The model under review builds one solid part; all positions refer to its coordinate system, in mm. A direction names the side the tool comes from. Coordinates: 2 decimals unless noted, no trailing zeros. Loops run counter-clockwise (first coordinate to the right, second up) from the corner with the lowest first, then second, coordinate; pieces in that order, holes last. Notation, with made-up numbers: (18, -4) - (54, -4) arc R17 ccw to (54, 28) - close; hole circle Ø11 at (-2.75, 30.25). An arc over 180 degrees is marked (long way). Answer in a Markdown table with one row per item. Add a question column.
(1) We need section B-B on y = 0.45. Write out the cut boundary in (x, z), plus the area to 3 significant figures.
(2) Mouldability with a two-part tool opening along X and no side actions: class faces 5 (the flat face through (20.41, 0.02, 18.64)), 6 (the flat face through (20.15, 3, -11)), 7 (the flat face through (0, -1.25, 0)) as +X half, -X half, draft (parallel to the pull), parting line (faces both ways), or undercut.
(3) We need section A-A on z = -8.7. Write out the cut boundary in (x, y), plus the area to 3 significant figures.
(4) Machinability: for faces 1 (the flat face through (15, 3, -12)), 2 (the flat face through (-16, 3, 14.5)), 3 (the flat face through (19, 3, -7)), 4 (the flat face through (-20.3, 0.02, 18.53)), which of the approach directions +Z, -Z, +X, -X, +Y, -Y give a long, thin tool a straight path to every point of the face, cutting with its end or side? Answer none if there is none.
(5) For line 1 along X through (y, z) = (1.65, -8.7); line 2 along Z through (x, y) = (-14.35, 0.25); line 3 along Z through (x, y) = (3.75, -0.3), list the stretches that pass through material, from the lowest coordinate up.
(6) We need section C-C on x = -5.5. Write out the cut boundary in (y, z).
(7) We need section D-D on x = -22. Write out the cut boundary in (y, z), plus the area to 3 significant figures.
(8) For P1, Ø1.8, axis at y = 3.5, z = 10.5, coming from the +X side; P2, Ø1, axis at y = 3.5, z = 10.5, coming from the -X side; P3, Ø6.5, axis at x = -15, z = -9.5, coming from the +Y side, all flat-tipped, find the tip position at first contact; note any pin that passes through.
from build123d import *

# Parameters (mm, degrees)
SKETCH3_W            = 55.2
SKETCH3_H            = 45
BOSS_EXTRUDE1_DEPTH  = 1.25
SKETCH4_R            = 4
BOSS_EXTRUDE2_DEPTH  = 2
M3_CLEARANCE_HOLE1_D = 3.4
BOSS_EXTRUDE3_DEPTH  = 3.5
CUT_EXTRUDE1_DEPTH   = 36.780721066
CIRPATTERN1_COUNT    = 4


with BuildPart() as part:
    # Sketch3 → Boss-Extrude1 (new, symmetric)
    with BuildSketch(Plane(origin=(0, 0, 0), x_dir=(1, 0, 0), z_dir=(0, 1, 0))):
        Rectangle(SKETCH3_W, SKETCH3_H)
    extrude(amount=BOSS_EXTRUDE1_DEPTH, both=True)

    # Sketch4 → Boss-Extrude2 (add)
    with BuildSketch(Plane(origin=(0, 1.25, 0), x_dir=(1, 0, 0), z_dir=(0, 1, 0))):
        with Locations(Location((-14.35, 8.7, 0), (0, 0, 90))):
            Circle(SKETCH4_R)
        with Locations(Location((3.75, -8.7, 0), (0, 0, 90))):
            Circle(SKETCH4_R)
    extrude(amount=BOSS_EXTRUDE2_DEPTH)

    # M3 Clearance Hole1 (through all)
    with Locations(Plane(origin=(0, 3.25, 0), x_dir=(1, 0, 0), z_dir=(0, 1, 0))):
        with Locations((-14.35, 8.7), (3.75, -8.7)):
            Hole(M3_CLEARANCE_HOLE1_D / 2)

    # Sketch7 → Boss-Extrude3 (add)
    with BuildSketch(Plane(origin=(0, 1.25, 0), x_dir=(1, 0, 0), z_dir=(0, 1, 0))):
        Polygon((-17.65, -12), (-17.65, -7), (-20.15, -7), (-20.15, -14.5), (-12.65, -14.5), (-12.65, -12), align=None)
        Polygon((17.65, 12), (12.65, 12), (12.65, 14.5), (20.15, 14.5), (20.15, 7), (17.65, 7), align=None)
    extrude(amount=BOSS_EXTRUDE3_DEPTH)

    # Sketch8 → Cut-Extrude1 (cut, symmetric)
    with BuildSketch(Plane(origin=(0, 1.25, 0), x_dir=(1, 0, 0), z_dir=(0, 1, 0))):
        Polygon((-30.32753429, 28.559767337), (-16.440232663, 14.67246571), (-14.67246571, 16.440232663), (-28.559767337, 30.32753429), align=None)
    cut_extrude1 = extrude(amount=CUT_EXTRUDE1_DEPTH, both=True, mode=Mode.SUBTRACT)

    # CirPattern1: Cut-Extrude1 ×4 about axis
    cirpattern1_axis = Axis((0, 0, 0), (0, 1, 0))
    for i in range(1, CIRPATTERN1_COUNT):
        add(cut_extrude1.rotate(cirpattern1_axis, i * 360 / CIRPATTERN1_COUNT), mode=Mode.SUBTRACT)


solid = part.part
Outcome:
| question | item | result |
|---|---|---|
| 1 | outline | (-27.6, -22.5) - (-24.27, -22.5) - (-16.44, -14.67) - (-14.67, -16.44) - (-20.73, -22.5) - (20.73, -22.5) - (14.67, -16.44) - (16.44, -14.67) - (24.27, -22.5) - (27.6, -22.5) - (27.6, 22.5) - (24.27, 22.5) - (16.44, 14.67) - (14.67, 16.44) - (20.73, 22.5) - (-20.73, 22.5) - (-14.67, 16.44) - (-16.44, 14.67) - (-24.27, 22.5) - (-27.6, 22.5) - close; hole circle Ø3.4 at (-14.35, -8.7); hole circle Ø3.4 at (3.75, 8.7) |
| 1 | area | 2,370 mm² |
| 2 | face 5 | undercut |
| 2 | face 6 | +X half |
| 2 | face 7 | draft |
| 3 | outline | (-27.6, -1.25) - (-16.05, -1.25) - (-16.05, 3.25) - (-18.35, 3.25) - (-18.35, 1.25) - (-27.6, 1.25) - close; (-12.65, -1.25) - (27.6, -1.25) - (27.6, 1.25) - (20.15, 1.25) - (20.15, 4.75) - (17.65, 4.75) - (17.65, 1.25) - (-10.35, 1.25) - (-10.35, 3.25) - (-12.65, 3.25) - close |
| 3 | area | 147 mm² |
| 4 | face 1 | +Z, +Y |
| 4 | face 2 | +Z, +X, -X, +Y |
| 4 | face 3 | +Z, +X, +Y |
| 4 | face 4 | +Y, -Y |
| 5 | line 1 | -18.35 to -16.05, -12.65 to -10.35, 17.65 to 20.15 |
| 5 | line 2 | -22.5 to -10.4, -7 to 22.5 |
| 5 | line 3 | -22.5 to 7, 10.4 to 22.5 |
| 6 | outline | (-1.25, -22.5) - (1.25, -22.5) - (1.25, 22.5) - (-1.25, 22.5) - close |
| 7 | outline | (-1.25, -20.23) - (1.25, -20.23) - (1.25, 20.23) - (-1.25, 20.23) - close |
| 7 | area | 101 mm² |
| 8 | P1 | x = 7.64 |
| 8 | P2 | x = -20.15 |
| 8 | P3 | y = 3.25 |
